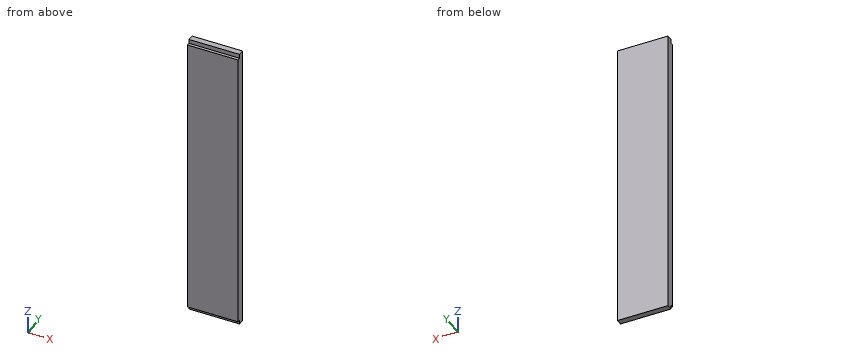
Autodesk Inventor part; units mm, degrees
ref_plane "YZ Plane" through (0, 0, 0) normal (1, 0, 0) x (0, 1, 0)
ref_plane "XZ Plane" through (0, 0, 0) normal (0, 1, 0) x (-1, 0, 0)
ref_plane "XY Plane" through (0, 0, 0) normal (0, 0, 1) x (1, 0, 0)
sketch "Sketch1" plane through (0, 0, 0) normal (0, 1, 0) x (-1, 0, 0)
  line L0 (28.3692, 74.6141) -> (-56.6308, 74.6141)
  line L1 (-56.6308, 74.6141) -> (-56.6308, -415.3859)
  line L2 (-56.6308, -415.3859) -> (28.3692, -415.3859)
  line L3 (28.3692, -415.3859) -> (28.3692, 74.6141)
  point P0 (0, 0)
  dimension "d0" = 85
  dimension "d1" = 490
extrude "Extrusion1" add sketch "Sketch1" along normal blind 15
sketch "Sketch2" plane through (-28.3692, 0, 74.6141) normal (0, 0, 1) x (1, 0, 0)
  line L0 (85, 0) -> (0, 0)
  line L1 (0, 0) -> (85, 0)
  line L2 (85, 0) -> (85, 5)
  line L3 (85, 5) -> (0, 5)
  line L4 (0, 5) -> (0, 0)
  point P0 (28.3692, 0)
  dimension "d4" = 85
  dimension "d5" = 5
extrude "Extrusion2" cut sketch "Sketch2" against normal blind 7
sketch "Sketch3" plane through (56.6308, 0, -415.3859) normal (0, 0, -1) x (-1, 0, 0)
  line L0 (85, 0) -> (85, 15)
  line L1 (85, 5) -> (0, 5)
  line L2 (85, 0) -> (0, 0)
  line L3 (0, 0) -> (0, 5)
  line L4 (0, 5) -> (85, 5)
  line L5 (85, 5) -> (85, 0)
  point P0 (56.6308, 0)
  dimension "d8" = 85
  dimension "d9" = 5
extrude "Extrusion3" cut sketch "Sketch3" against normal blind 7
properties part number "Arcade_top"
The model under review builds one solid part; all positions refer to its coordinate system, in mm. Give positions to 0.01 mm unless a question says otherwise; leave off trailing zeros. Write each loop counter-clockwise with the first axis right and the second up, starting at its lowest first coordinate (ties: lowest second). Pieces come first, ordered by that corner, then holes.
1. Wall thickness on L1, parallel to Z at x = 22.5, y = 1.25: over which ranges is the line inside the solid? List them lowest first.
2. For P1, Ø1.5, axis at x = 5.5, y = 2, coming from the +Z side; P2, Ø5.5, axis at x = 0, z = -413, coming from the -Y side; P3, Ø1.5, axis at x = 34.5, y = 3.5, coming from the -Z side, all flat-tipped, find the tip position at first contact; note any pin that passes through.
3. Add section A-A, the plane y = 2.5. Write out the cut boundary in (x, z).
Worked answers:
1. L1: z = -408.39 to 67.61
2. P1: stops at z = 67.61
2. P2: stops at y = 5
2. P3: stops at z = -408.39
3. outline: (-28.37, -408.39) - (56.63, -408.39) - (56.63, 67.61) - (-28.37, 67.61) - close
